Here's how the part is built. I have some questions about the finished solid (model axes, mm). Round coordinates to 2 decimals unless told otherwise and drop trailing zeros. Use a Markdown table: item, result.
```python
from build123d import *

# Parameters (mm, degrees)
SKETCH_1_W          = 150
SKETCH_1_H          = 45.5
EXTRUDE_1_DEPTH     = 2
CUT_EXTRUDE_1_REACH = 80.4
SKETCH_2_R          = 1.65
CUT_EXTRUDE_2_REACH = 80.4
SKETCH_4_W          = 10
SKETCH_4_H          = 5
CHAMFER_1_SIZE      = 8
SKETCH_6_W          = 14.5
SKETCH_6_H          = 32.5
EXTRUDE_2_DEPTH     = 2
CUT_EXTRUDE_3_REACH = 94.368
SKETCH_7_R          = 1.65
CHAMFER_2_SIZE      = 5


with BuildPart() as part:
    # Sketch 1 → Extrude 1 (new body)
    with BuildSketch(Plane(origin=(0, 0, 0), x_dir=(1, 0, 0), z_dir=(0, 1, 0))):
        Rectangle(SKETCH_1_W, SKETCH_1_H)
    extrude(amount=EXTRUDE_1_DEPTH)

    # Sketch 2 → Cut-Extrude 1 (cut, up to next)
    with BuildSketch(Plane(origin=(0, 2, 0), x_dir=(1, 0, 0), z_dir=(0, 1, 0)), mode=Mode.PRIVATE) as cut_extrude_1_sk1:
        with Locations(Location((-60, 15, 0), (0, 0, 270))):
            Circle(SKETCH_2_R)
    cut_extrude_1_tool1 = extrude(cut_extrude_1_sk1.sketch, amount=-CUT_EXTRUDE_1_REACH, mode=Mode.PRIVATE) & part.part
    # Sketch 2 → Cut-Extrude 1 (cut, up to next)
    with BuildSketch(Plane(origin=(0, 2, 0), x_dir=(1, 0, 0), z_dir=(0, 1, 0)), mode=Mode.PRIVATE) as cut_extrude_1_sk2:
        with Locations(Location((-66, 7, 0), (0, 0, 270))):
            Circle(SKETCH_2_R)
    cut_extrude_1_tool2 = extrude(cut_extrude_1_sk2.sketch, amount=-CUT_EXTRUDE_1_REACH, mode=Mode.PRIVATE) & part.part
    # Sketch 2 → Cut-Extrude 1 (cut, up to next)
    with BuildSketch(Plane(origin=(0, 2, 0), x_dir=(1, 0, 0), z_dir=(0, 1, 0)), mode=Mode.PRIVATE) as cut_extrude_1_sk3:
        with Locations(Location((-54, 7, 0), (0, 0, 270))):
            Circle(SKETCH_2_R)
    cut_extrude_1_tool3 = extrude(cut_extrude_1_sk3.sketch, amount=-CUT_EXTRUDE_1_REACH, mode=Mode.PRIVATE) & part.part
    # Sketch 2 → Cut-Extrude 1 (cut, up to next)
    with BuildSketch(Plane(origin=(0, 2, 0), x_dir=(1, 0, 0), z_dir=(0, 1, 0)), mode=Mode.PRIVATE) as cut_extrude_1_sk4:
        with Locations(Location((-71, -7, 0), (0, 0, 270))):
            Circle(SKETCH_2_R)
    cut_extrude_1_tool4 = extrude(cut_extrude_1_sk4.sketch, amount=-CUT_EXTRUDE_1_REACH, mode=Mode.PRIVATE) & part.part
    # Sketch 2 → Cut-Extrude 1 (cut, up to next)
    with BuildSketch(Plane(origin=(0, 2, 0), x_dir=(1, 0, 0), z_dir=(0, 1, 0)), mode=Mode.PRIVATE) as cut_extrude_1_sk5:
        with Locations(Location((-59, -7, 0), (0, 0, 270))):
            Circle(SKETCH_2_R)
    cut_extrude_1_tool5 = extrude(cut_extrude_1_sk5.sketch, amount=-CUT_EXTRUDE_1_REACH, mode=Mode.PRIVATE) & part.part
    # Sketch 2 → Cut-Extrude 1 (cut, up to next)
    with BuildSketch(Plane(origin=(0, 2, 0), x_dir=(1, 0, 0), z_dir=(0, 1, 0)), mode=Mode.PRIVATE) as cut_extrude_1_sk6:
        with Locations(Location((-65, -15, 0), (0, 0, 270))):
            Circle(SKETCH_2_R)
    cut_extrude_1_tool6 = extrude(cut_extrude_1_sk6.sketch, amount=-CUT_EXTRUDE_1_REACH, mode=Mode.PRIVATE) & part.part
    cut_extrude_1_1 = cut_extrude_1_tool1.solids().sort_by_distance((-60, 2, -15))[0]
    add(cut_extrude_1_1, mode=Mode.SUBTRACT)
    cut_extrude_1_2 = cut_extrude_1_tool2.solids().sort_by_distance((-66, 2, -7))[0]
    add(cut_extrude_1_2, mode=Mode.SUBTRACT)
    cut_extrude_1_3 = cut_extrude_1_tool3.solids().sort_by_distance((-54, 2, -7))[0]
    add(cut_extrude_1_3, mode=Mode.SUBTRACT)
    cut_extrude_1_4 = cut_extrude_1_tool4.solids().sort_by_distance((-71, 2, 7))[0]
    add(cut_extrude_1_4, mode=Mode.SUBTRACT)
    cut_extrude_1_5 = cut_extrude_1_tool5.solids().sort_by_distance((-59, 2, 7))[0]
    add(cut_extrude_1_5, mode=Mode.SUBTRACT)
    cut_extrude_1_6 = cut_extrude_1_tool6.solids().sort_by_distance((-65, 2, 15))[0]
    add(cut_extrude_1_6, mode=Mode.SUBTRACT)
    cut_extrude_1 = cut_extrude_1_1 + cut_extrude_1_2 + cut_extrude_1_3 + cut_extrude_1_4 + cut_extrude_1_5 + cut_extrude_1_6  # Cut-Extrude 1 as one shape, for the pattern or mirror that repeats it

    # Sketch 4 → Cut-Extrude 2 (cut, up to next)
    with BuildSketch(Plane(origin=(0, 2, 0), x_dir=(1, 0, 0), z_dir=(0, 1, 0)), mode=Mode.PRIVATE) as cut_extrude_2_sk1:
        with Locations((-43, -20.25)):
            Rectangle(SKETCH_4_W, SKETCH_4_H)
    cut_extrude_2_tool1 = extrude(cut_extrude_2_sk1.sketch, amount=-CUT_EXTRUDE_2_REACH, mode=Mode.PRIVATE) & part.part
    cut_extrude_2 = cut_extrude_2_tool1.solids().sort_by_distance((-43, 2, 20.25))[0]
    add(cut_extrude_2, mode=Mode.SUBTRACT)

    # Mirror 1: Cut-Extrude 1, Cut-Extrude 2 across plane
    add(cut_extrude_1.mirror(Plane(origin=(0, 0, 0), x_dir=(0, 0, 1), z_dir=(1, 0, 0))), mode=Mode.SUBTRACT)
    add(cut_extrude_2.mirror(Plane(origin=(0, 0, 0), x_dir=(0, 0, 1), z_dir=(1, 0, 0))), mode=Mode.SUBTRACT)

    # Chamfer 1
    chamfer_1_edges = [part.edges().sort_by_distance(p)[0] for p in [
        (75, 1, 22.75),
        (-75, 1, 22.75),
    ]]
    chamfer(chamfer_1_edges, length=CHAMFER_1_SIZE)

    # Sketch 6 → Extrude 2 (add)
    with BuildSketch(Plane(origin=(0, 0, 0), x_dir=(1, 0, 0), z_dir=(0, 1, 0))):
        with Locations((-82.25, 1.5)):
            Rectangle(SKETCH_6_W, SKETCH_6_H)
    extrude_2 = extrude(amount=EXTRUDE_2_DEPTH)

    # Sketch 7 → Cut-Extrude 3 (cut, up to next)
    with BuildSketch(Plane(origin=(0, 2, 0), x_dir=(1, 0, 0), z_dir=(0, 1, 0)), mode=Mode.PRIVATE) as cut_extrude_3_sk1:
        with Locations(Location((-86, -8.5, 0), (0, 0, 270))):
            Circle(SKETCH_7_R)
    cut_extrude_3_tool1 = extrude(cut_extrude_3_sk1.sketch, amount=-CUT_EXTRUDE_3_REACH, mode=Mode.PRIVATE) & part.part
    # Sketch 7 → Cut-Extrude 3 (cut, up to next)
    with BuildSketch(Plane(origin=(0, 2, 0), x_dir=(1, 0, 0), z_dir=(0, 1, 0)), mode=Mode.PRIVATE) as cut_extrude_3_sk2:
        with Locations(Location((-86, 11.5, 0), (0, 0, 270))):
            Circle(SKETCH_7_R)
    cut_extrude_3_tool2 = extrude(cut_extrude_3_sk2.sketch, amount=-CUT_EXTRUDE_3_REACH, mode=Mode.PRIVATE) & part.part
    # Sketch 7 → Cut-Extrude 3 (cut, up to next)
    with BuildSketch(Plane(origin=(0, 2, 0), x_dir=(1, 0, 0), z_dir=(0, 1, 0)), mode=Mode.PRIVATE) as cut_extrude_3_sk3:
        with Locations(Location((-39, -11.5, 0), (0, 0, 270))):
            Circle(SKETCH_7_R)
    cut_extrude_3_tool3 = extrude(cut_extrude_3_sk3.sketch, amount=-CUT_EXTRUDE_3_REACH, mode=Mode.PRIVATE) & part.part
    # Sketch 7 → Cut-Extrude 3 (cut, up to next)
    with BuildSketch(Plane(origin=(0, 2, 0), x_dir=(1, 0, 0), z_dir=(0, 1, 0)), mode=Mode.PRIVATE) as cut_extrude_3_sk4:
        with Locations(Location((-39, 8.5, 0), (0, 0, 270))):
            Circle(SKETCH_7_R)
    cut_extrude_3_tool4 = extrude(cut_extrude_3_sk4.sketch, amount=-CUT_EXTRUDE_3_REACH, mode=Mode.PRIVATE) & part.part
    cut_extrude_3_1 = cut_extrude_3_tool1.solids().sort_by_distance((-86, 2, 8.5))[0]
    add(cut_extrude_3_1, mode=Mode.SUBTRACT)
    cut_extrude_3_2 = cut_extrude_3_tool2.solids().sort_by_distance((-86, 2, -11.5))[0]
    add(cut_extrude_3_2, mode=Mode.SUBTRACT)
    cut_extrude_3_3 = cut_extrude_3_tool3.solids().sort_by_distance((-39, 2, 11.5))[0]
    add(cut_extrude_3_3, mode=Mode.SUBTRACT)
    cut_extrude_3_4 = cut_extrude_3_tool4.solids().sort_by_distance((-39, 2, -8.5))[0]
    add(cut_extrude_3_4, mode=Mode.SUBTRACT)
    cut_extrude_3 = cut_extrude_3_1 + cut_extrude_3_2 + cut_extrude_3_3 + cut_extrude_3_4  # Cut-Extrude 3 as one shape, for the pattern or mirror that repeats it

    # Mirror 3: Extrude 2, Cut-Extrude 3 across plane
    add(extrude_2.mirror(Plane(origin=(0, 0, 0), x_dir=(0, 0, 1), z_dir=(1, 0, 0))))
    add(cut_extrude_3.mirror(Plane(origin=(0, 0, 0), x_dir=(0, 0, 1), z_dir=(1, 0, 0))), mode=Mode.SUBTRACT)

    # Chamfer 2
    chamfer_2_edges = [part.edges().sort_by_distance(p)[0] for p in [
        (-75, 1, -17.75),
        (75, 1, -17.75),
    ]]
    chamfer(chamfer_2_edges, length=CHAMFER_2_SIZE - 0.0001)  # a hair under: the kernel refuses the full size


solid = part.part
```
Q1. We'd pull the mould along X, two halves only. Please class faces 1 (the flat face through (-70.94, 0.99, 18.81)), 2 (the flat face through (70.94, 0.99, 18.81)), 3 (the cylindrical face through (66.6, 1, 14.6)): pulls with the +X half, pulls with the -X half, needs draft (parallel to the pull), parting line crosses it, or undercut.
Return value:
| item | result |
|---|---|
| face 1 | pulls with the -X half |
| face 2 | pulls with the +X half |
| face 3 | undercut |
Q2. Imagine slicing it at A-A, the plane y = 1.55. Give the number of separate pieces and of enclosed holes in the cut face, then the cut area to 3 significant figures.
Return value:
| item | result |
|---|---|
| separate pieces | 1 |
| enclosed holes | 20 |
| area | 7,460 mm^2 |
Q3. I need wall thicknesses on line 1 (Z direction, x = 39, y = 0.2); line 2 (X direction, y = 1.2, z = 15); line 3 (X direction, y = 0.9, z = 10.5). Which ranges of each line are inside material? Lowest first, please. Write a range as from..to.
Return value:
| item | result |
|---|---|
| line 1 | z = -22.75..-10.15, -6.85..9.85, 13.15..17.75 |
| line 2 | x = -74.75..-66.65, -63.35..63.35, 66.65..74.75 |
| line 3 | x = -89.5..-40.31, -37.69..37.69, 40.31..89.5 |
Q4. Will these pins go through, and if not, where does the flat tip stop? P1, Ø0.6, axis at x = -83.5, y = 1, coming from the +Z side; P2, Ø2, axis at x = 39, z = 11.5, coming from the -Y side; P3, Ø1, axis at y = 0.5, z = 21, coming from the +X side; P4, Ø1, axis at y = 1.5, z = 21, coming from the -X side.
Return value:
| item | result |
|---|---|
| P1 | stops at z = 14.75 |
| P2 | passes through |
| P3 | stops at x = 69.25 |
| P4 | stops at x = -69.25 |
